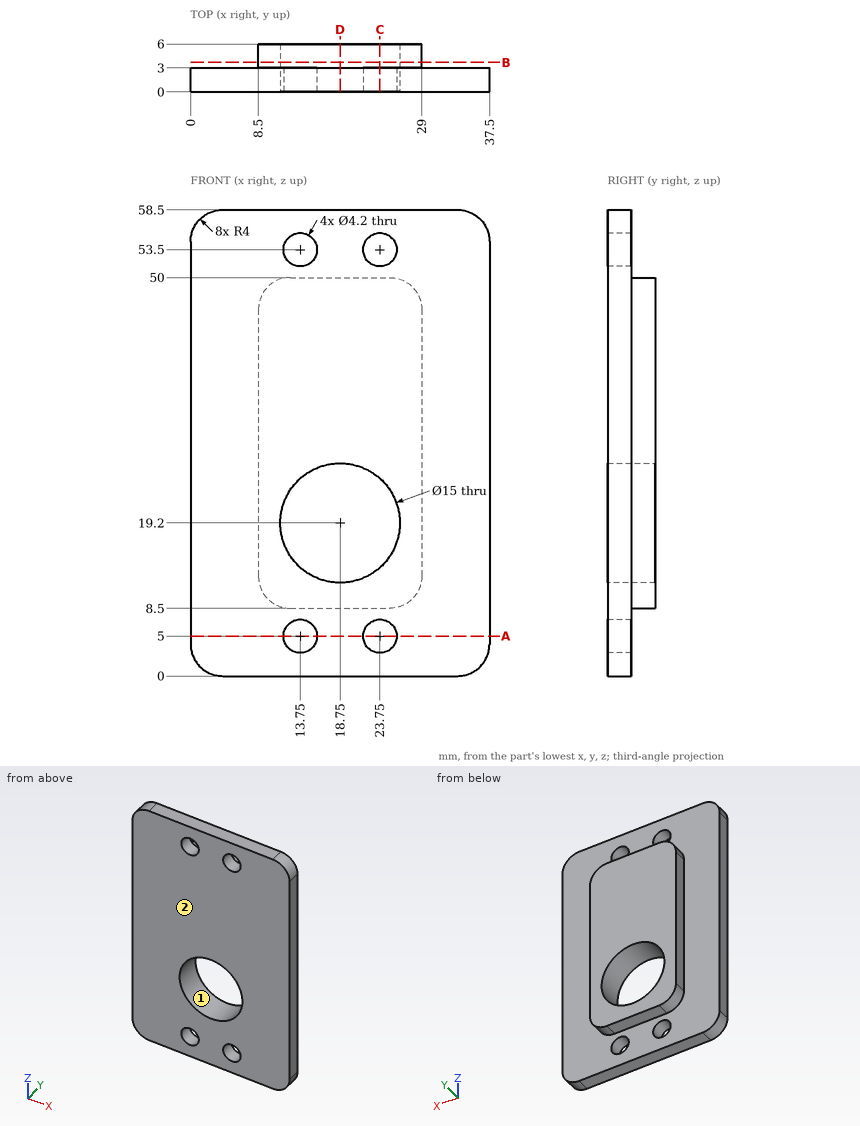
Check sheet for the drawn part. Datum: minimum x, y, z corner. Units: mm. Give positions to 0.01 mm unless a question says otherwise; leave off trailing zeros. Order: outer loops, then holes, each group sorted by start corner. A loop starts at its lowest first (then second) coordinate and runs counter-clockwise, first axis right, second up. Notation, with made-up numbers: (65.25, -8) - (118.25, -8) arc R13 ccw to (118.25, 10) - close; hole circle Ø3 at (-2.5, 39). An arc over 180 degrees is marked (long way). Answer as a JSON object with one key per item and string values.
(1) Cross-section at B-B (y = 3.7). Record the cut outline in (x, z), then the cut area to 3 significant figures.
Report:
{"outline": "(8.5, 12.5) arc R4 ccw to (12.5, 8.5) - (25, 8.5) arc R4 ccw to (29, 12.5) - (29, 46) arc R4 ccw to (25, 50) - (12.5, 50) arc R4 ccw to (8.5, 46) - close; hole circle Ø15 at (18.75, 19.2)", "area": "660 mm^2"}
(2) Material ranges on line 1 (X direction, y = 1.9, z = 53.5); line 2 (X direction, y = 2.05, z = 19.2); line 3 (Y direction, x = 32, z = 15.5), recorded low to high.
Report:
{"line 1": "0 to 11.65, 15.85 to 21.65, 25.85 to 37.5", "line 2": "0 to 11.25, 26.25 to 37.5", "line 3": "0 to 3"}
(3) Depth check by flat-ended pin: pin 1 Ø3.5 at (y, z) = (5, 33) entering from +X; pin 2 Ø2.5 at (x, z) = (23.75, 5) entering from -Y; pin 3 Ø2.5 at (x, y) = (21, 5) entering from -Z; pin 4 Ø3 at (x, y) = (29.5, 5) entering from +Z. Enter the tip coordinate at first touch or a pass-through.
Report:
{"pin 1": "x = 29", "pin 2": "through", "pin 3": "z = 8.5", "pin 4": "z = 48.65"}
(4) Draft check along Z on the marked faces 1 and 2. Enter one of: released by +Z, released by -Z, zero draft, split by the parting line, or undercut.
Report:
{"face 1": "undercut", "face 2": "zero draft"}
(5) Cross-section at D-D (x = 18.75). Record the cut outline in (y, z), then the cut area to 3 significant figures.
Report:
{"outline": "(0, 0) - (3, 0) - (3, 8.5) - (6, 8.5) - (6, 11.7) - (0, 11.7) - close; (0, 26.7) - (6, 26.7) - (6, 50) - (3, 50) - (3, 58.5) - (0, 58.5) - close", "area": "210 mm^2"}
(6) Cross-section at C-C (x = 23.75). Record the cut outline in (y, z).
Report:
{"outline": "(0, 0) - (3, 0) - (3, 2.9) - (0, 2.9) - close; (0, 7.1) - (3, 7.1) - (3, 8.5) - (6, 8.5) - (6, 13.61) - (0, 13.61) - close; (0, 24.79) - (6, 24.79) - (6, 50) - (3, 50) - (3, 51.4) - (0, 51.4) - close; (0, 55.6) - (3, 55.6) - (3, 58.5) - (0, 58.5) - close"}
(7) Cross-section at A-A (z = 5). Record the cut outline in (x, y).
Report:
{"outline": "(0, 0) - (11.65, 0) - (11.65, 3) - (0, 3) - close; (15.85, 0) - (21.65, 0) - (21.65, 3) - (15.85, 3) - close; (25.85, 0) - (37.5, 0) - (37.5, 3) - (25.85, 3) - close"}
